from build123d import *

# Parameters (mm, degrees)
KES_EKSTR_ZYON1_DEPTH = 431
IZIM3_W               = 1.6
IZIM3_H               = 0.7
KES_EKSTR_ZYON2_DEPTH = 5


with BuildPart() as part:
    # Çizim1 → Döndür1 (revolve)
    with BuildSketch(Plane.XY, mode=Mode.PRIVATE) as d_nd_r1_sk:
        Polygon((-325.5, 0), (325.5, 0), (325.5, 15), (245.5, 15), (245.5, 17.5), (-185.5, 17.5), (-185.5, 15), (-325.5, 15), align=None)
    revolve(d_nd_r1_sk.sketch.rotate(Axis((-325.5, 0, 0), (1, 0, 0)), 90), axis=Axis((-325.5, 0, 0), (1, 0, 0)))

    # Çizim2 → Kes-Ekstrüzyon1 (cut)
    with BuildSketch(Plane.ZY.offset(185.5)):
        with BuildLine():
            Line((-14.843898339, 9.268693657), (-15.15172785, -8.756434386))
            ThreePointArc((-15.15172785, -8.756434386), (-17.49744861, 0.298817908), (-14.843898339, 9.268693657))
        make_face()
        with BuildLine():
            Line((14.843898339, 9.268693657), (15.15172785, -8.756434386))
            ThreePointArc((15.15172785, -8.756434386), (17.49744861, 0.298817908), (14.843898339, 9.268693657))
        make_face()
    extrude(amount=-KES_EKSTR_ZYON1_DEPTH, mode=Mode.SUBTRACT)

    # Çizim3 → Kes-Döndür2 (revolve, cut)
    with BuildSketch(Plane(origin=(0, 0, 0), x_dir=(1, 0, 0), z_dir=(0, 1, 0)), mode=Mode.PRIVATE) as kes_d_nd_r2_sk:
        with Locations((-321.7, 14.65)):
            Rectangle(IZIM3_W, IZIM3_H)
    revolve(kes_d_nd_r2_sk.sketch.rotate(Axis((-325.5, 0, 0), (1, 0, 0)), 180), axis=Axis((-325.5, 0, 0), (1, 0, 0)), mode=Mode.SUBTRACT)

    # Çizim6 → Kes-Ekstrüzyon2 (cut)
    with BuildSketch(Plane(origin=(0, -11.490666647, 9.641814145), x_dir=(0, -0.642787609686535, -0.7660444431189818), z_dir=(0, 0.7660444431189817, -0.6427876096865349))):
        with BuildLine():
            Line((5, 312.5), (5, 272.5))
            ThreePointArc((5, 272.5), (0, 267.5), (-5, 272.5))
            Line((-5, 272.5), (-5, 312.5))
            ThreePointArc((-5, 312.5), (0, 317.5), (5, 312.5))
        make_face()
    extrude(amount=KES_EKSTR_ZYON2_DEPTH, mode=Mode.SUBTRACT)


solid = part.part
Here's how the part is built. I have some questions about the finished solid (model axes, mm). A direction names the side the tool comes from. Coordinates: 2 decimals unless noted, no trailing zeros. Loops run counter-clockwise (first coordinate to the right, second up) from the corner with the lowest first, then second, coordinate; pieces in that order, holes last. Notation, with made-up numbers: (44, -36) -> (99, -36) arc R20 ccw to (99, -15) -> close; hole circle Ø4 at (85, 32.25). An arc over 180 degrees is marked (long way). Use one line per item in the form item = value. Start each with the question number.
(1) If we section it at B-B (x = 67.5): Please give me the cut outline in (y, z).
(2) If we section it at A-A (x = -280): Please give me the cut outline in (y, z), then the cut area to 3 significant figures.
(3) Please list where these lines run through material, in increasing order: line 1 along Z through (x, y) = (-212.5, -1); line 2 along X through (y, z) = (-8, -12.5); line 3 along X through (y, z) = (-13, 8.5).
(4) Will these pins go through, and if not, where does the flat tip stop? pin 1 (4 mm diameter, centred on x = -46, y = -6.5, fed in from +Z); pin 2 (5 mm diameter, centred on x = -106, y = 9.5, fed in from -Z); pin 3 (1.5 mm diameter, centred on x = 260, y = -5, fed in from -Z).
(5) On a 3-axis mill with a long thin cutter (end or side, diameter ignored), from which of +Z, -Z, +X, -X, +Y, -Y can I reach the whole of each face in a straight line? I mean faces 1 (the face through (245.5, 15.2, 1.2)), 2 (the face through (-185.5, -15.2, -0.1)), 3 (the face through (-324.02, -12.65, 8.06)). Say none if no direction works.
(6) We'd pull the mould along X, two halves only. Please class faces 4 (the face through (-321.69, -14.18, -1.86)), 5 (the face through (-185.5, 15.2, -1.2)), 6 (the face through (26.98, -17.5, 0.26)), 7 (the face through (325.5, 0, 0)): pulls with the +X half, pulls with the -X half, needs draft (parallel to the pull), parting line crosses it, or undercut.
Verdict:
q1.outline = (-8.76, -15.15) -> (9.27, -14.84) arc R17.5 ccw to (9.27, 14.84) -> (-8.76, 15.15) arc R17.5 ccw to start
q2.outline = (-14.05, 5.26) arc R15 ccw (long way) to (-7.62, 12.92) -> (-4.45, 10.26) -> (-10.87, 2.6) -> close
q2.area = 660 mm²
q3.line_1 = -14.97 to 14.97
q3.line_2 = -325.5 to -322.5, -320.9 to 325.5
q3.line_3 = -185.5 to 245.5
q4.pin_1 = 15.15
q4.pin_2 = -14.88
q4.pin_3 = -14.39
q5.face_1 = +X, +Y
q5.face_2 = -X, -Y
q5.face_3 = -X
q6.face_4 = undercut
q6.face_5 = pulls with the -X half
q6.face_6 = needs draft
q6.face_7 = pulls with the +X half
